from build123d import *

# Parameters (mm, degrees)
SKETCH_1_W          = 43
SKETCH_1_H          = 43
EXTRUDE_1_DEPTH     = 4
FILLET_1_R          = 3.5
SKETCH_2_R          = 1.75
CUT_EXTRUDE_1_DEPTH = 31.66757245
SKETCH_3_R          = 6
EXTRUDE_2_DEPTH     = 6
SKETCH_4_R          = 3
EXTRUDE_3_DEPTH     = 15
CUT_EXTRUDE_START   = -12
CUT_EXTRUDE_2_DEPTH = 12
SKETCH_6_R          = 19
EXTRUDE_4_DEPTH     = 21.5
SKETCH_7_R          = 16
EXTRUDE_5_DEPTH     = 29


with BuildPart() as part:
    # 스케치1 → 보스-돌출1 (new body)
    with BuildSketch(Plane.XY):
        Rectangle(SKETCH_1_W, SKETCH_1_H)
    extrude(amount=EXTRUDE_1_DEPTH)

    # 필렛1
    fillet_1_edges = [part.edges().sort_by_distance(p)[0] for p in [
        (21.5, -21.5, 2),
        (-21.5, -21.5, 2),
        (-21.5, 21.5, 2),
        (21.5, 21.5, 2),
    ]]
    fillet(fillet_1_edges, radius=FILLET_1_R)

    # 스케치2 → 컷-돌출1 (cut, through all)
    with BuildSketch(Plane.XY.offset(4)):
        with Locations((18, 18)):
            Circle(SKETCH_2_R)
        with Locations(Location((-18, 18, 0), (0, 0, 180))):
            Circle(SKETCH_2_R)
        with Locations(Location((18, -18, 0), (0, 0, 180))):
            Circle(SKETCH_2_R)
        with Locations((-18, -18)):
            Circle(SKETCH_2_R)
    extrude(amount=-CUT_EXTRUDE_1_DEPTH, mode=Mode.SUBTRACT)

    # 스케치3 → 보스-돌출2 (add)
    with BuildSketch(Plane.XY.offset(4)):
        with Locations(Location((0, 7, 0), (0, 0, 180))):
            Circle(SKETCH_3_R)
    extrude(amount=EXTRUDE_2_DEPTH)

    # 스케치4 → 보스-돌출3 (add)
    with BuildSketch(Plane.XY.offset(10)):
        with Locations((0, 7)):
            Circle(SKETCH_4_R)
    extrude(amount=EXTRUDE_3_DEPTH)

    # 스케치5 → 컷-돌출2 (cut)
    with BuildSketch(Plane.XY.offset(25).offset(CUT_EXTRUDE_START)):
        with BuildLine():
            Line((-1.658312395, 9.5), (1.658312395, 9.5))
            ThreePointArc((1.658312395, 9.5), (0, 10), (-1.658312395, 9.5))
        make_face()
    extrude(amount=CUT_EXTRUDE_2_DEPTH, mode=Mode.SUBTRACT)

    # 스케치6 → 보스-돌출4 (add)
    with BuildSketch(Plane(origin=(0, 0, 0), x_dir=(-1, 0, 0), z_dir=(0, 0, -1))):
        Circle(SKETCH_6_R)
    extrude(amount=EXTRUDE_4_DEPTH)

    # 스케치7 → 보스-돌출5 (add)
    with BuildSketch(Plane(origin=(0, 0, -21.5), x_dir=(-1, 0, 0), z_dir=(0, 0, -1))):
        with Locations(Location((0, 0, 0), (0, 0, 180))):
            Circle(SKETCH_7_R)
    extrude(amount=EXTRUDE_5_DEPTH)


solid = part.part
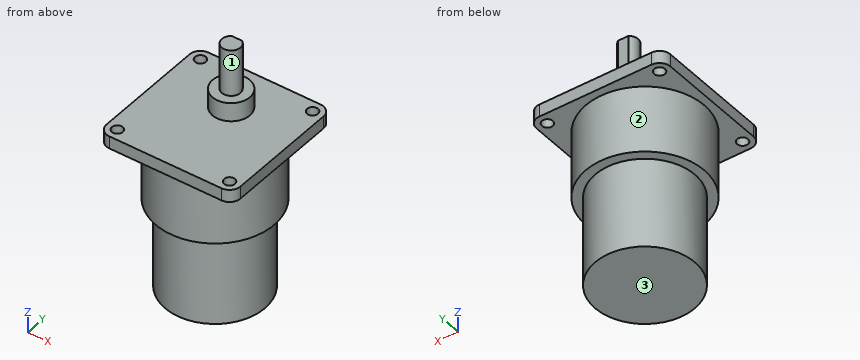
The model under review builds one solid part; all positions refer to its coordinate system, in mm. Face numbers are marked on the shaded views. A direction names the side the tool comes from. Give positions to 0.01 mm unless a question says otherwise; leave off trailing zeros. Order: outer loops, then holes, each group sorted by start corner. A loop starts at its lowest first (then second) coordinate and runs counter-clockwise, first axis right, second up. Notation, with made-up numbers: M 6.5,63 L 62.5,63 A16 ccw 62.5,76 Z; hole C 34.25,-20 d10. An arc over 180 degrees is marked long. Answer in a Markdown table with one row per item. Add a question column.
1. Add section B-B on y = -2.5. State the section outline as (x, z) points, plus the area to 3 significant figures.
2. Machinability: for the marked faces 1, 2 and 3, which of the approach directions +Z, -Z, +X, -X, +Y, -Y give a long, thin tool a straight path to every point of the face, cutting with its end or side? Answer none if there is none.
3. To check wall thickness, follow line 1 along Y through (x, z) = (-18, 1.5); line 2 along Z through (x, y) = (-17, -3); line 3 along Z through (x, y) = (-10, -10). State the ranges of each line that lie inside material, in increasing order.
4. For pin 1 Ø4 at (x, y) = (8.5, -5.5) entering from +Z; pin 2 Ø2.5 at (x, z) = (0.5, 16.5) entering from +Y; pin 3 Ø8 at (x, z) = (-3, 9.5) entering from -Y, all flat-tipped, find the tip position at first contact; note any pin that passes through.
5. Add section C-C on z = -43. State the section outline as (x, y) points.
6. Add section A-A on x = 0. State the section outline as (y, z) points, plus the area to 3 significant figures.
7. Add section D-D on y = 7. State the section outline as (x, z) points.
The answers:
| question | item | result |
|---|---|---|
| 1 | outline | M -21.5,0 L -18.83,0 L -18.83,-21.5 L -15.8,-21.5 L -15.8,-50.5 L 15.8,-50.5 L 15.8,-21.5 L 18.83,-21.5 L 18.83,0 L 21.5,0 L 21.5,4 L -21.5,4 Z |
| 1 | area | 1,900 mm2 |
| 2 | face 1 | +Z |
| 2 | face 2 | -Z |
| 2 | face 3 | -Z, +X, -X, +Y, -Y |
| 3 | line 1 | -21.5 to -19.75, -16.25 to 16.25, 19.75 to 21.5 |
| 3 | line 2 | -21.5 to 4 |
| 3 | line 3 | -50.5 to 4 |
| 4 | pin 1 | z = 4 |
| 4 | pin 2 | y = 9.5 |
| 4 | pin 3 | y = 1 |
| 5 | outline | C 0,0 d32 |
| 6 | outline | M -21.5,0 L -19,0 L -19,-21.5 L -16,-21.5 L -16,-50.5 L 16,-50.5 L 16,-21.5 L 19,-21.5 L 19,0 L 21.5,0 L 21.5,4 L 13,4 L 13,10 L 10,10 L 10,13 L 9.5,13 L 9.5,25 L 4,25 L 4,10 L 1,10 L 1,4 L -21.5,4 Z |
| 6 | area | 2,070 mm2 |
| 7 | outline | M -21.5,0 L -17.66,0 L -17.66,-21.5 L -14.39,-21.5 L -14.39,-50.5 L 14.39,-50.5 L 14.39,-21.5 L 17.66,-21.5 L 17.66,0 L 21.5,0 L 21.5,4 L 6,4 L 6,10 L 3,10 L 3,25 L -3,25 L -3,10 L -6,10 L -6,4 L -21.5,4 Z |
